Input: part model. Units: mm. Frame: model coordinates. A direction names the side the tool comes from. Give positions to 0.01 mm unless a question says otherwise; leave off trailing zeros. Order: outer loops, then holes, each group sorted by start corner. A loop starts at its lowest first (then second) coordinate and runs counter-clockwise, first axis right, second up.
```python
from build123d import *

# Parameters (mm, degrees)
F0_R      = 10
F0_R_2    = 2
F1_DEPTH  = 2
F2_R      = 10
F2_R_2    = 8
F3_DEPTH  = 28
F4_R      = 10.5
F4_R_2    = 8
F5_DEPTH  = 1
F6_R      = 10
F6_R_2    = 8
F7_DEPTH  = 1
F8_R      = 10.5
F8_R_2    = 8
F9_DEPTH  = 1
F10_R     = 10
F10_R_2   = 8
F11_DEPTH = 1
F12_R     = 10.5
F12_R_2   = 8
F13_DEPTH = 1


with BuildPart() as f1:
    # F0 (on Top) → F1 (new body)
    with BuildSketch(Plane.XY):
        Circle(F0_R)
        Circle(F0_R_2, mode=Mode.SUBTRACT)
    extrude(amount=F1_DEPTH)

    # F2 (on face) → F3 (join)
    with BuildSketch(Plane.XY.offset(2)):
        Circle(F2_R)
        Circle(F2_R_2, mode=Mode.SUBTRACT)
    extrude(amount=F3_DEPTH)

    # F4 (on face) → F5 (join)
    with BuildSketch(Plane.XY.offset(30)):
        Circle(F4_R)
        Circle(F4_R_2, mode=Mode.SUBTRACT)
    extrude(amount=F5_DEPTH)

    # F6 (on face) → F7 (join)
    with BuildSketch(Plane.XY.offset(31)):
        Circle(F6_R)
        Circle(F6_R_2, mode=Mode.SUBTRACT)
    extrude(amount=F7_DEPTH)

    # F8 (on face) → F9 (join)
    with BuildSketch(Plane.XY.offset(32)):
        Circle(F8_R)
        Circle(F8_R_2, mode=Mode.SUBTRACT)
    extrude(amount=F9_DEPTH)

    # F10 (on face) → F11 (join)
    with BuildSketch(Plane.XY.offset(33)):
        Circle(F10_R)
        Circle(F10_R_2, mode=Mode.SUBTRACT)
    extrude(amount=F11_DEPTH)

    # F12 (on face) → F13 (join)
    with BuildSketch(Plane.XY.offset(34)):
        Circle(F12_R)
        Circle(F12_R_2, mode=Mode.SUBTRACT)
    extrude(amount=F13_DEPTH)


solid = f1.part
```
1) Pull-direction query (Y, two-part tool) for faces 1 (the face through (2, -2, 2)), 2 (the face through (-2.17, -9.76, 33.49)), 3 (the face through (5, -9, 31)); classes: pulls with the +Y half, pulls with the -Y half, needs draft (parallel to the pull), parting line crosses it, or undercut.
2) Line query: probe 1 along Z at (x, y) = (9.5, 3.5); probe 2 along X at (y, z) = (-0.25, 3.5). Output: solid intervals per line, ascending.
3) Cut plane C-C (z = 20.5). Return the cut outline in (x, y).
4) First-contact query: P1, Ø8, axis at y = 5.5, z = 6, coming from the +X side; P2, Ø3, axis at y = -5.5, z = 26.5, coming from the -X side; P3, Ø4, axis at y = 3, z = 23.5, coming from the -X side. Flat tips, straight axial feed; report the tip coordinate or a pass-through.
5) Cut plane D-D (y = -9). Return the cut outline in (x, z), then the cut area to 3 significant figures.
6) Reachability of faces 4 (the face through (0, -2, 1)), 5 (the face through (-2.17, -9.76, 14.79)), 6 (the face through (-2, -8, 35)), 7 (the face through (-1.73, -7.81, 18.27)), 8 (the face through (5, -9, 33)) from +Z, -Z, +X, -X, +Y, -Y: full face, straight path, thin tool, end or side. Return the list, or none.
Geometry says:
1. face 1: undercut
1. face 2: parting line crosses it
1. face 3: needs draft
2. probe 1: z = 30 to 31, 32 to 33, 34 to 35
2. probe 2: x = -10 to -8, 8 to 10
3. outline: circle Ø20 at (0, 0); hole circle Ø16 at (0, 0)
4. P1: stops at x = 9.89
4. P2: stops at x = -9.17
4. P3: stops at x = -9.95
5. outline: (-5.41, 30) - (-4.36, 30) - (-4.36, 0) - (4.36, 0) - (4.36, 30) - (5.41, 30) - (5.41, 31) - (4.36, 31) - (4.36, 32) - (5.41, 32) - (5.41, 33) - (4.36, 33) - (4.36, 34) - (5.41, 34) - (5.41, 35) - (-5.41, 35) - (-5.41, 34) - (-4.36, 34) - (-4.36, 33) - (-5.41, 33) - (-5.41, 32) - (-4.36, 32) - (-4.36, 31) - (-5.41, 31) - close
5. area: 311 mm2
6. face 4: +Z, -Z
6. face 5: -Z
6. face 6: +Z, +X, -X, +Y, -Y
6. face 7: +Z
6. face 8: none
